from build123d import *

# Parameters (mm, degrees)
F1_DEPTH = 52
F4_R     = 11
F5_DEPTH = 44.7
F6_R     = 25.99999


# Not quite as in the source:
# - a fillet or chamfer is up to 0.001 mm smaller than in the source, because OpenCascade refuses the exact size


with BuildPart() as f1:
    # F0 (on Top) → F1 (new body)
    with BuildSketch(Plane.XY):
        with BuildLine():
            ThreePointArc((-42, 0), (0, 42), (42, 0))
            Line((42, 0), (182, 0))
            Line((182, 0), (182, 38))
            Line((182, 38), (62.329768169, 38))
            ThreePointArc((62.329768169, 38), (-19.7348286497, 70.2818364741), (-73, 0))
            Line((-73, 0), (-42, 0))
        make_face()
    extrude(amount=F1_DEPTH)

    # F2 (on face) → F3 (revolve, cut)
    with BuildSketch(Plane.XZ):
        Polygon((0, 0), (0, 52), (-60, 52), (-42, 0), align=None)
    revolve(axis=Axis((0, 0, 26), (0, 0, -1)), mode=Mode.SUBTRACT)

    # F4 (on face) → F5 (cut)
    with BuildSketch(Plane.XZ):
        with Locations((108, 26)):
            Circle(F4_R)
        with Locations((156, 26)):
            Circle(F4_R)
    extrude(amount=-F5_DEPTH, mode=Mode.SUBTRACT)

    # F6 (radius 26 in the source; OpenCascade refuses exactly that, so slightly less here)
    f6_edges = [f1.edges().sort_by_distance(p)[0] for p in [
        (182, 19, 52),
        (182, 19, 0),
    ]]
    fillet(f6_edges, radius=F6_R)


solid = f1.part
Verification items for the finished model (mm, model axes). A direction names the side the tool comes from. Round coordinates to 2 decimals unless told otherwise and drop trailing zeros. Order: outer loops, then holes, each group sorted by start corner. A loop starts at its lowest first (then second) coordinate and runs counter-clockwise, first axis right, second up.
1. Access from +Z, -Z, +X, -X, +Y, -Y to the whole of each face (thin tool, end or side, straight path). Record for faces 4 (the flat face through (65, 29, 52)), 5 (the flat face through (123, 38, 26)).
Final values:
face 4: +Z, +X, -X, +Y, -Y
face 5: +Z, -Z, +X, +Y
2. Release check for a two-part mould opening along Z. For faces 1 (the flat face through (40, 29, 0)), 2 (the cylindrical face through (145, 19, 26)), 3 (the cylindrical face through (-18.455, 70.629, 25.636)) record: +Z half, -Z half, draft (parallel to the pull), parting line (faces both ways), or undercut.
Final values:
face 1: -Z half
face 2: undercut
face 3: draft
3. Go/stop test with flat-tipped pins: P1, Ø1.5, axis at y = 27.5, z = 8, coming from the -X side; P2, Ø5, axis at y = 18, z = 28, coming from the -X side; P3, Ø2, axis at y = 15.5, z = 33.5, coming from the +X side. Record where each tip stops, or that it passes through.
Final values:
P1: stops at x = -67.92
P2: stops at x = -71.34
P3: stops at x = 181.17
4. Section check A-A on x = 108. Record the cut outline in (y, z).
Final values:
outline: (0, 0) - (38, 0) - (38, 15) - (0, 15) - close; (0, 37) - (38, 37) - (38, 52) - (0, 52) - close
5. Section check C-C on y = 33. State how many separate pieces and enclosed holes the cut face has, then the cut area to 3 significant figures.
Final values:
separate pieces: 2
enclosed holes: 2
area: 7,780 mm2
6. Thickness scan on L1, parallel to Z at x = 108, y = 26.5; L2, parallel to X at y = 27.5, z = 31; L3, parallel to X at y = 8, z = 32. Record the ranges inside material, lowest first.
Final values:
L1: z = 0 to 15, 37 to 52
L2: x = -67.62 to -44.99, 44.99 to 98.2, 117.8 to 146.2, 165.8 to 181.51
L3: x = -72.56 to -52.47, 52.47 to 98.78, 117.22 to 146.78, 165.22 to 181.3
7. Section check B-B on z = 20. Record the cut outline in (x, y).
Final values:
outline: (-73, 0) - (-48.92, 0) arc R48.92 cw to (48.92, 0) - (98.78, 0) - (98.78, 38) - (62.33, 38) arc R73 ccw to start; (117.22, 0) - (146.78, 0) - (146.78, 38) - (117.22, 38) - close; (165.22, 0) - (181.3, 0) - (181.3, 38) - (165.22, 38) - close
8. Section check D-D on x = 0. Record the cut outline in (y, z).
Final values:
outline: (42, 0) - (73, 0) - (73, 52) - (60, 52) - close
